Source: CAD feature listing. Evaluate the final solid. Frame: model axes, mm. A direction names the side the tool comes from. Give positions to 0.01 mm unless a question says otherwise; leave off trailing zeros. Order: outer loops, then holes, each group sorted by start corner. A loop starts at its lowest first (then second) coordinate and runs counter-clockwise, first axis right, second up. Notation, with made-up numbers: M 35.5,-29 L 91.5,-29 A7 ccw 91.5,-21 Z; hole C 25,2.25 d7. An arc over 180 degrees is marked long. Return JSON: item names as keys, results as strings.
from build123d import *

# Parameters (mm, degrees)
ESBO_O1_W                  = 180
ESBO_O1_H                  = 65
RESSALTO_EXTRUS_O3_DEPTH   = 32.5
FILETE6_R                  = 33
CORTE_EXTRUS_O2_DEPTH      = 116.677353013
CORTE_EXTRUS_O2_DEPTH_BACK = 116.677353013
ESBO_O5_W                  = 65
ESBO_O5_H                  = 35
FILETE7_R                  = 33
CORTE_EXTRUS_O3_DEPTH      = 116.674405799
CORTE_EXTRUS_O3_DEPTH_BACK = 116.674405799
ESBO_O8_W                  = 65
ESBO_O8_H                  = 35
CORTE_EXTRUS_O4_DEPTH      = 116.674405799
CORTE_EXTRUS_O4_DEPTH_BACK = 116.674405799
ESBO_O11_R                 = 10


with BuildPart() as part:
    # Esboço1 → Ressalto-extrusão3 (new, symmetric)
    with BuildSketch(Plane(origin=(0, 0, 0), x_dir=(1, 0, 0), z_dir=(0, 1, 0))):
        Rectangle(ESBO_O1_W, ESBO_O1_H)
    extrude(amount=RESSALTO_EXTRUS_O3_DEPTH, both=True)

    # Filete6
    # the kernel refuses this fillet: 33 mm, written as the material it takes off along each edge
    with BuildSketch(Plane(origin=(90, 115, -32.5), x_dir=(-1, 0, 0), z_dir=(0, -1, 0))) as filete6_piece_1:
        with BuildLine():
            CenterArc((FILETE6_R, -FILETE6_R), FILETE6_R, 90, 90)
            Line((0, -FILETE6_R), (0, 0))
            Line((0, 0), (FILETE6_R, 0))
        make_face()
    extrude(amount=230, mode=Mode.SUBTRACT)
    with BuildSketch(Plane(origin=(90, 115, 32.5), x_dir=(-1, 0, 0), z_dir=(0, -1, 0))) as filete6_piece_2:
        with BuildLine():
            CenterArc((FILETE6_R, FILETE6_R), FILETE6_R, 180, 90)
            Line((0, FILETE6_R), (0, 0))
            Line((0, 0), (FILETE6_R, 0))
        make_face()
    extrude(amount=230, mode=Mode.SUBTRACT)

    # Esboço5 → Corte-extrusão2 (cut, two sides: drawn at the far end of the back side and taken through both)
    with BuildSketch(Plane.XY.offset(32.5).offset(-CORTE_EXTRUS_O2_DEPTH_BACK)):
        with Locations((57.496211904, 0)):
            Rectangle(ESBO_O5_W, ESBO_O5_H)
    extrude(amount=CORTE_EXTRUS_O2_DEPTH + CORTE_EXTRUS_O2_DEPTH_BACK, mode=Mode.SUBTRACT)

    # Filete7
    # the kernel refuses this fillet: 33 mm, written as the material it takes off along each edge
    with BuildSketch(Plane(origin=(-90, -32.5, 115), x_dir=(0, 1, 0), z_dir=(0, 0, -1))) as filete7_piece_1:
        with BuildLine():
            CenterArc((FILETE7_R, FILETE7_R), FILETE7_R, 180, 90)
            Line((0, FILETE7_R), (0, 0))
            Line((0, 0), (FILETE7_R, 0))
        make_face()
    extrude(amount=230, mode=Mode.SUBTRACT)
    with BuildSketch(Plane(origin=(-90, 32.5, 115), x_dir=(0, -1, 0), z_dir=(0, 0, -1))) as filete7_piece_2:
        with BuildLine():
            CenterArc((FILETE7_R, -FILETE7_R), FILETE7_R, 90, 90)
            Line((0, -FILETE7_R), (0, 0))
            Line((0, 0), (FILETE7_R, 0))
        make_face()
    extrude(amount=230, mode=Mode.SUBTRACT)

    # Esboço8 → Corte-extrusão3 (cut, two sides: drawn at the far end of the back side and taken through both)
    with BuildSketch(Plane(origin=(0, 32.5, 0), x_dir=(1, 0, 0), z_dir=(0, 1, 0)).offset(-CORTE_EXTRUS_O3_DEPTH_BACK)):
        with Locations((-57.496211904, 0)):
            Rectangle(ESBO_O8_W, ESBO_O8_H)
    extrude(amount=CORTE_EXTRUS_O3_DEPTH + CORTE_EXTRUS_O3_DEPTH_BACK, mode=Mode.SUBTRACT)

    # Esboço11 → Corte-extrusão4 (cut, two sides: drawn at the far end of the back side and taken through both)
    with BuildSketch(Plane(origin=(0, 32.5, 0), x_dir=(1, 0, 0), z_dir=(0, 1, 0)).offset(-CORTE_EXTRUS_O4_DEPTH_BACK)):
        with Locations(Location((59.485722432, 0, 0), (0, 0, 270))):
            Circle(ESBO_O11_R)
    extrude(amount=CORTE_EXTRUS_O4_DEPTH + CORTE_EXTRUS_O4_DEPTH_BACK, mode=Mode.SUBTRACT)


solid = part.part
1. Section query B-B (z = -5.5). Return loops of the section in (x, y), then the cut area to 3 significant figures.
Evaluation:
{"outline": "M -25,-32.5 L 51.13,-32.5 L 51.13,-17.5 L 25,-17.5 L 25,17.5 L 51.13,17.5 L 51.13,32.5 L -25,32.5 Z; M 67.84,-32.5 L 89.45,-32.5 L 89.45,-17.5 L 67.84,-17.5 Z; M 67.84,17.5 L 89.45,17.5 L 89.45,32.5 L 67.84,32.5 Z", "area": "4,680 mm^2"}
2. Section query D-D (x = -62). Return loops of the section in (y, z), then the cut area to 3 significant figures.
Evaluation:
{"outline": "M -32.12,-32.5 L 32.12,-32.5 L 32.12,-17.5 L -32.12,-17.5 Z; M -32.12,17.5 L 32.12,17.5 L 32.12,32.5 L -32.12,32.5 Z", "area": "1,930 mm^2"}
3. First-contact query: pin 1 (5 mm diameter, centred on y = 17.5, z = -18, fed in from -X); pin 2 (1 mm diameter, centred on y = 20.5, z = -7.5, fed in from +X); pin 3 (10.5 mm diameter, centred on y = 2, z = 10, fed in from +X). Flat tips, straight axial feed; report the tip coordinate or a pass-through.
Evaluation:
{"pin 1": "stops at x = -86.13", "pin 2": "stops at x = 89.14", "pin 3": "stops at x = 25"}
4. Section query A-A (x = -27). Return loops of the section in (y, z).
Evaluation:
{"outline": "M -32.5,-32.5 L 32.5,-32.5 L 32.5,-17.5 L -32.5,-17.5 Z; M -32.5,17.5 L 32.5,17.5 L 32.5,32.5 L -32.5,32.5 Z"}
5. Draft query along Z for faces 1 (the face through (-80.41, 22.76, 25.11)), 2 (the face through (80.41, 25.11, 22.76)), 3 (the face through (79.9, 25.11, -23.26)), 4 (the face through (49.724, -25.105, -2.168)). Return one class per face: pulls with the +Z half, pulls with the -Z half, needs draft (parallel to the pull), parting line crosses it, or undercut.
Evaluation:
{"face 1": "needs draft", "face 2": "pulls with the +Z half", "face 3": "pulls with the -Z half", "face 4": "undercut"}
6. Ray query, probe 1 along Z at (x, y) = (-32, 18); probe 2 along X at (y, z) = (22.5, 0). Return the intervals inside material, ascending.
Evaluation:
{"probe 1": "z = -32.5 to -17.5, 17.5 to 32.5", "probe 2": "x = -25 to 49.49, 69.49 to 90"}
7. Set-up query: faces 5 (the face through (50, 17.5, 7)), 6 (the face through (-80.41, 22.76, -24.9)), 7 (the face through (-24.996, 0, 0)). Return all of +Z, -Z, +X, -X, +Y, -Y with unobstructed straight access to the full face (end or side cutting, diameter ignored); none if empty.
Evaluation:
{"face 5": "+Z, -Z, +X", "face 6": "+Z, -Z, -X, +Y", "face 7": "-X, +Y, -Y"}
8. Section query C-C (y = -21). Return loops of the section in (x, z).
Evaluation:
{"outline": "M -82.03,-32.5 L 57,-32.5 A33 ccw 90,0 A33 ccw 57,32.5 L -82.03,32.5 L -82.03,17.5 L -25,17.5 L -25,-17.5 L -82.03,-17.5 Z; hole C 59.49,0 d20"}
